Here's the drawing with two shaded views (mm, measured from the low corner). I have some questions. A direction names the side the tool comes from. Round coordinates to 2 decimals unless told otherwise and drop trailing zeros. Write each loop counter-clockwise with the first axis right and the second up, starting at its lowest first coordinate (ties: lowest second). Pieces come first, ordered by that corner, then holes. Notation, with made-up numbers: (-21.5, -3) - (11.5, -3) arc R32 ccw to (11.5, 24) - close; hole circle Ø11 at (-30, 59). An arc over 180 degrees is marked (long way). Return JSON: item names as keys, results as strings. Group by question number.
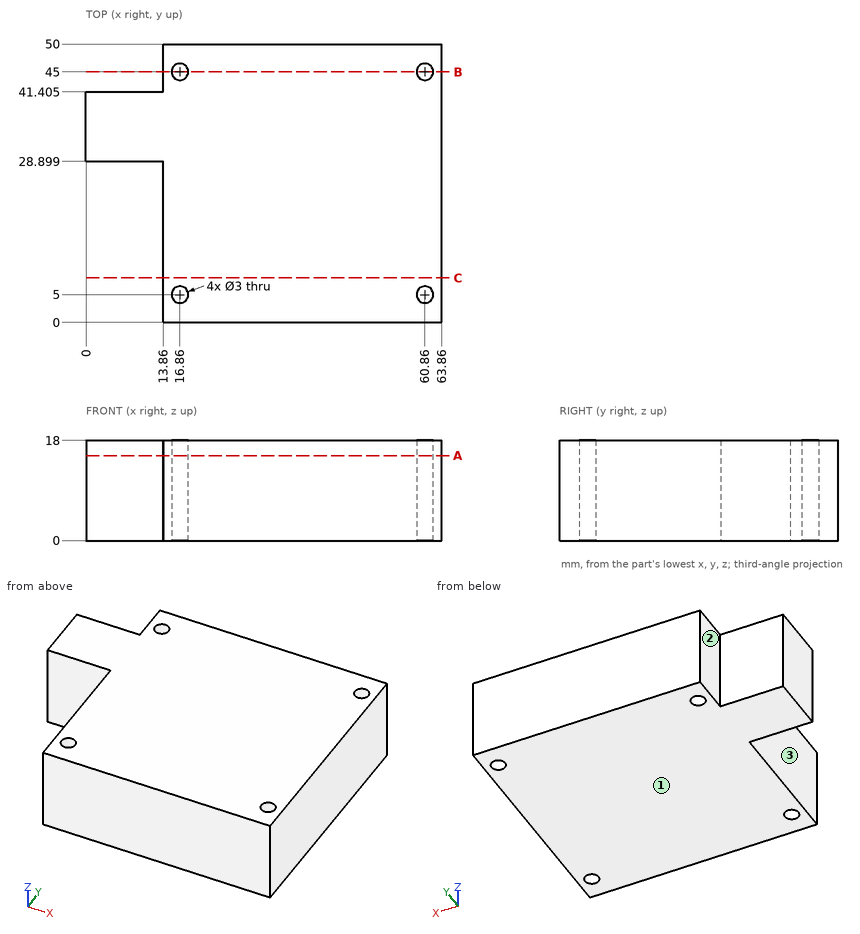
1) Imagine slicing it at A-A (z = 15.25). Please give me the cut outline in (x, y) (1 decimal), plus the area to 4 significant figures.
2) Imagine slicing it at C-C (y = 8). Please give me the cut outline in (x, z), plus the area to 3 significant figures.
3) For the marked faces 1, 2 and 3, which set-ups out of +Z, -Z, +X, -X, +Y, -Y let a thin tool reach every point of the face, with its end or its side?
4) Imagine slicing it at B-B (y = 45). Please give me the cut outline in (x, z), plus the area to 3 significant figures.
5) Will these pins go through, and if not, where does the flat tip stop? pin 1 Ø2.5 at (x, y) = (60.86, 5) entering from +Z; pin 2 Ø9 at (y, z) = (16.5, 13) entering from -X; pin 3 Ø4 at (x, z) = (8, 6.5) entering from +Y (1 decimal).
6) I need wall thicknesses on line 1 along X through (y, z) = (4, 16.25); line 2 along Y through (x, z) = (59.5, 9.75) (1 decimal); line 3 along X through (y, z) = (16, 14.75). Which ranges of each line are inside material? Lowest first, please.
Results found:
{
 "1": {"outline": "(0, 28.9) - (13.9, 28.9) - (13.9, 0) - (63.9, 0) - (63.9, 50) - (13.9, 50) - (13.9, 41.4) - (0, 41.4) - close; hole circle Ø3 at (16.9, 5); hole circle Ø3 at (16.9, 45); hole circle Ø3 at (60.9, 5); hole circle Ø3 at (60.9, 45)", "area": "2,645 mm²"},
 "2": {"outline": "(13.86, 0) - (63.86, 0) - (63.86, 18) - (13.86, 18) - close", "area": "900 mm²"},
 "3": {"face 1": "-Z, +X, -X, +Y, -Y", "face 2": "+Z, -Z, -X, +Y", "face 3": "+Z, -Z, -X, -Y"},
 "4": {"outline": "(13.86, 0) - (15.36, 0) - (15.36, 18) - (13.86, 18) - close; (18.36, 0) - (59.36, 0) - (59.36, 18) - (18.36, 18) - close; (62.36, 0) - (63.86, 0) - (63.86, 18) - (62.36, 18) - close", "area": "792 mm²"},
 "5": {"pin 1": "passes through", "pin 2": "stops at x = 13.86", "pin 3": "stops at y = 41.4"},
 "6": {"line 1": "x = 13.86 to 15.74, 17.98 to 59.74, 61.98 to 63.86", "line 2": "y = 0 to 4.4, 5.6 to 44.4, 45.6 to 50", "line 3": "x = 13.86 to 63.86"}
}
